For this review, use the dimensioned drawing (mm, ordinates from the lowest corner) and the shaded views. A direction names the side the tool comes from. Give positions to 0.01 mm unless a question says otherwise; leave off trailing zeros. Write each loop counter-clockwise with the first axis right and the second up, starting at its lowest first coordinate (ties: lowest second). Pieces come first, ordered by that corner, then holes.
1) Machinability: for the marked faces 1 and 2, which of the approach directions +Z, -Z, +X, -X, +Y, -Y give a long, thin tool a straight path to every point of the face, cutting with its end or side? Answer none if there is none.
2) Wall thickness on line 1 along Z through (x, y) = (18.5, 3); line 2 along Z through (x, y) = (10.5, 22.5); line 3 along Y through (x, z) = (6, 4.15): over which ranges is each line inside the solid? List them lowest first.
3) We need section D-D on x = 22.5. Give the boundary of the cut face in (y, z).
4) We need section A-A on x = 12. Give the boundary of the cut face in (y, z).
5) We need section C-C on z = 4.05. Give the boundary of the cut face in (x, y).
6) For P1, Ø3, axis at y = 7, z = 1.5, coming from the +X side, flat-tipped, find the tip position at first contact; note if it passes through.
7) We need section B-B on y = 5. Give the boundary of the cut face in (x, z), and give its area (3 significant figures).
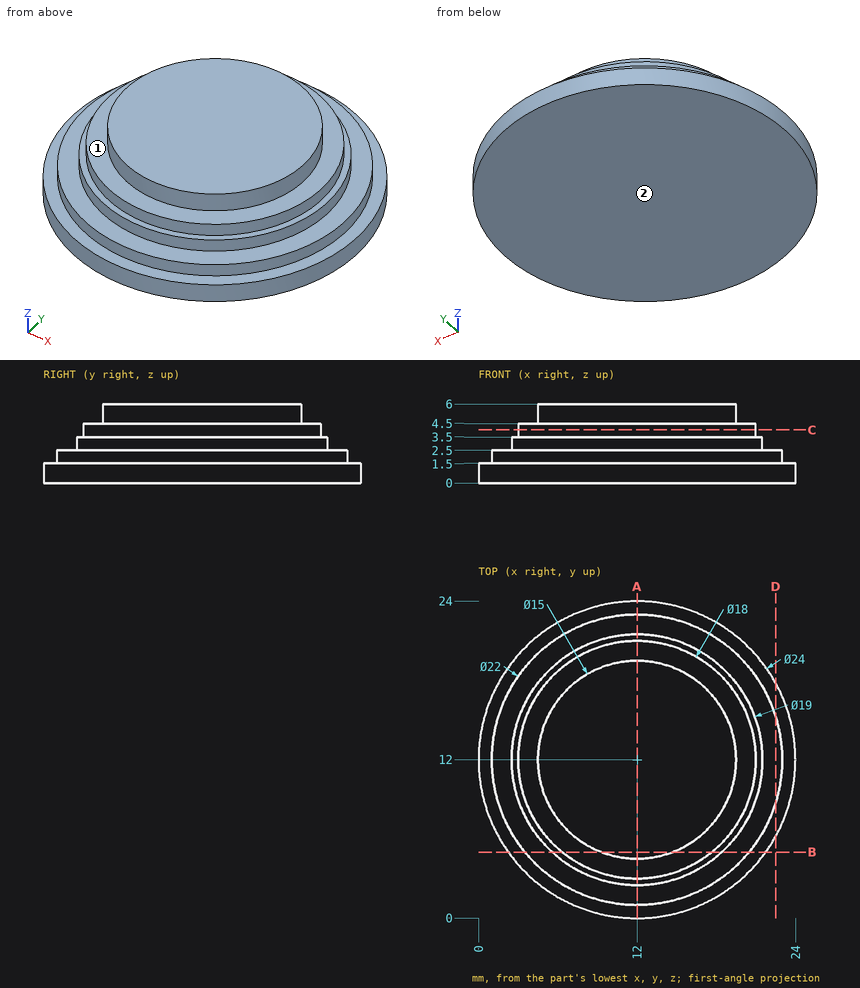
Results list:
1. face 1: +Z
1. face 2: -Z, +X, -X, +Y, -Y
2. line 1: z = 0 to 1.5
2. line 2: z = 0 to 2.5
2. line 3: y = 5.29 to 18.71
3. outline: (6.19, 0) - (17.81, 0) - (17.81, 1.5) - (15.28, 1.5) - (15.28, 2.5) - (8.72, 2.5) - (8.72, 1.5) - (6.19, 1.5) - close
4. outline: (0, 0) - (24, 0) - (24, 1.5) - (23, 1.5) - (23, 2.5) - (21.5, 2.5) - (21.5, 3.5) - (21, 3.5) - (21, 4.5) - (19.5, 4.5) - (19.5, 6) - (4.5, 6) - (4.5, 4.5) - (3, 4.5) - (3, 3.5) - (2.5, 3.5) - (2.5, 2.5) - (1, 2.5) - (1, 1.5) - (0, 1.5) - close
5. outline: circle Ø18 at (12, 12)
6. P1: stops at x = 23.48
7. outline: (2.25, 0) - (21.75, 0) - (21.75, 1.5) - (20.49, 1.5) - (20.49, 2.5) - (18.42, 2.5) - (18.42, 3.5) - (17.66, 3.5) - (17.66, 4.5) - (14.69, 4.5) - (14.69, 6) - (9.31, 6) - (9.31, 4.5) - (6.34, 4.5) - (6.34, 3.5) - (5.58, 3.5) - (5.58, 2.5) - (3.51, 2.5) - (3.51, 1.5) - (2.25, 1.5) - close
7. area: 78.4 mm2
